Job drawing, mm, ordinate dimensions from the low corner. One solid piece. A direction names the side the tool comes from. Give positions to 0.01 mm unless a question says otherwise; leave off trailing zeros. Order: outer loops, then holes, each group sorted by start corner. A loop starts at its lowest first (then second) coordinate and runs counter-clockwise, first axis right, second up.
1. Slice it at C-C on x = 17.75. List the corners of the cut face in (y, z).
2. Slice it at A-A on z = 15.5. List the corners of the cut face in (x, y), and give its area (3 significant figures).
3. Slice it at B-B on y = 60.5. List the corners of the cut face in (x, z).
4. Slice it at D-D on z = 22.25. List the corners of the cut face in (x, y).
5. Which spindle directions (+Z, -Z, +X, -X, +Y, -Y) get a long thin tool onto all of the face, cutting with end or side? Do the marked faces 1 and 2. Say none if no direction does.
6. Probe line 1 (Y direction, x = 12.5, z = 13); line 2 (Y direction, x = 4.25, z = 14.75). List the from-to ranges inside material, lowest first.
7. Drop flat-ended pins along their axis: pin 1 Ø10 at (x, z) = (12, 14) entering from +Y; pin 2 Ø12.5 at (y, z) = (49.5, 15.5) entering from +X. Give the stop position or say it passes through.
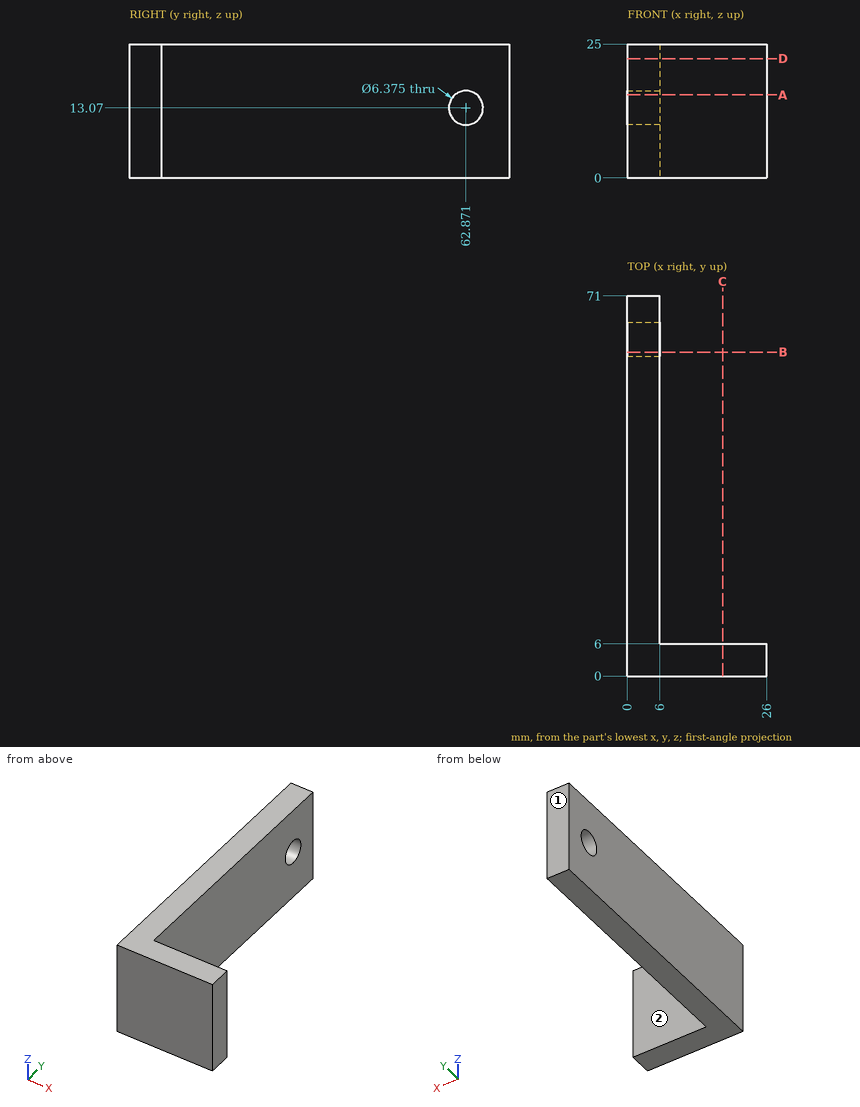
Data:
1. outline: (0, 0) - (6, 0) - (6, 25) - (0, 25) - close
2. outline: (0, 0) - (26, 0) - (26, 6) - (6, 6) - (6, 60.81) - (0, 60.81) - close; (0, 64.93) - (6, 64.93) - (6, 71) - (0, 71) - close
2. area: 521 mm2
3. outline: (0, 0) - (6, 0) - (6, 10.94) - (0, 10.94) - close; (0, 15.2) - (6, 15.2) - (6, 25) - (0, 25) - close
4. outline: (0, 0) - (26, 0) - (26, 6) - (6, 6) - (6, 71) - (0, 71) - close
5. face 1: +Z, -Z, +X, -X, +Y
5. face 2: +Z, -Z, +X, +Y
6. line 1: y = 0 to 6
6. line 2: y = 0 to 60.16, 65.58 to 71
7. pin 1: stops at y = 6
7. pin 2: stops at x = 6
